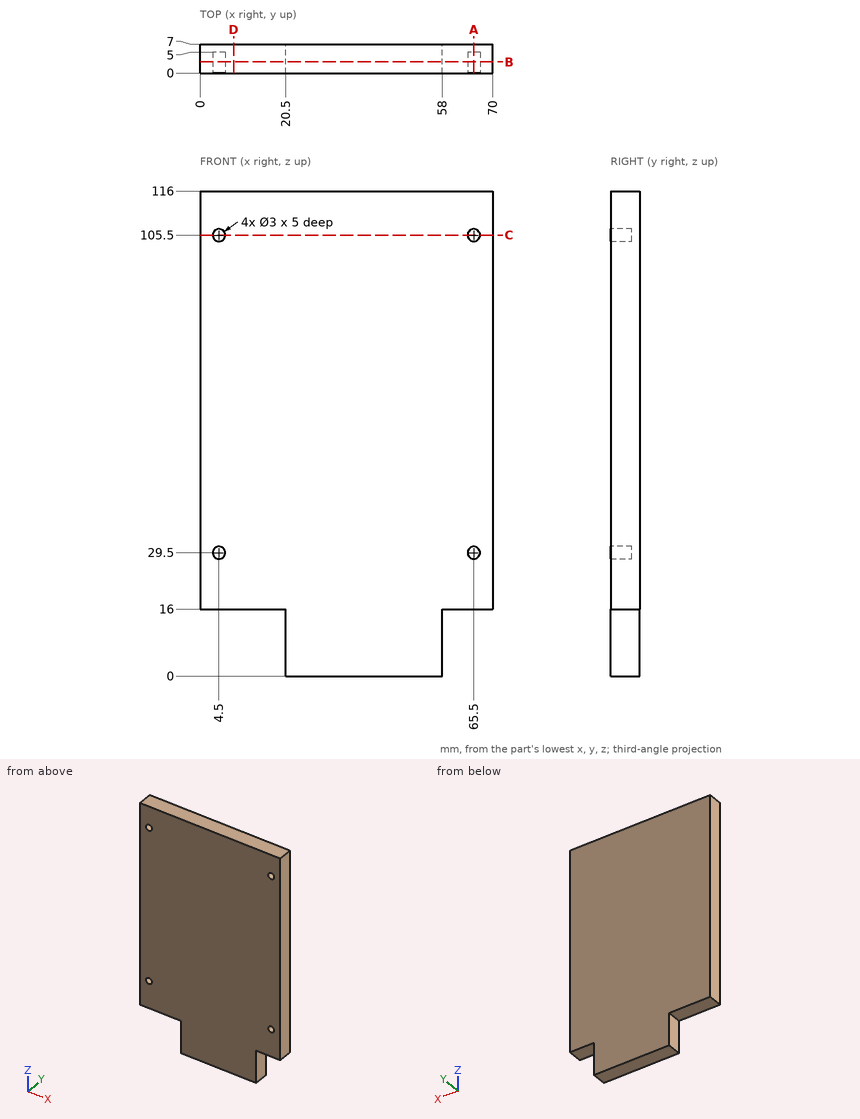
Could you check a few things on this drawing? It's one solid part, dimensions in mm from its lowest x, y, z. Coordinates: 2 decimals unless noted, no trailing zeros. Order: outer loops, then holes, each group sorted by start corner. A loop starts at its lowest first (then second) coordinate and runs counter-clockwise, first axis right, second up. Notation, with made-up numbers: (-34, 84) - (10, 84) arc R32 ccw to (10, 118) - close; hole circle Ø9 at (-16, -14.75). An arc over 180 degrees is marked (long way). One line per question, with ' | ' between items.
(1) If I drill on L1, parallel to X at y = 1.65, z = 29.5; L2, parallel to Z at x = 65.5, y = 3.05; L3, parallel to X at y = 3, z = 104.5, over which ranges is the centre line in solid material (lowest first)?
Report:
L1: x = 0 to 3, 6 to 64, 67 to 70 | L2: z = 16 to 28, 31 to 104, 107 to 116 | L3: x = 0 to 3.38, 5.62 to 64.38, 66.62 to 70
(2) Suppose I cut it at B-B on y = 2.75. List the corners of the cut face in (x, z) for me.
Report:
outline: (0, 16) - (20.5, 16) - (20.5, 0) - (58, 0) - (58, 16) - (70, 16) - (70, 116) - (0, 116) - close; hole circle Ø3 at (4.5, 29.5); hole circle Ø3 at (4.5, 105.5); hole circle Ø3 at (65.5, 29.5); hole circle Ø3 at (65.5, 105.5)
(3) Suppose I cut it at A-A on x = 65.5. List the corners of the cut face in (y, z) for me.
Report:
outline: (0, 16) - (7, 16) - (7, 116) - (0, 116) - (0, 107) - (5, 107) - (5, 104) - (0, 104) - (0, 31) - (5, 31) - (5, 28) - (0, 28) - close
(4) Suppose I cut it at C-C on z = 105.5. List the corners of the cut face in (x, y) for me, and give its area (3 significant figures).
Report:
outline: (0, 0) - (3, 0) - (3, 5) - (6, 5) - (6, 0) - (64, 0) - (64, 5) - (67, 5) - (67, 0) - (70, 0) - (70, 7) - (0, 7) - close | area: 460 mm2
(5) Suppose I cut it at D-D on x = 8. List the corners of the cut face in (y, z) for me.
Report:
outline: (0, 16) - (7, 16) - (7, 116) - (0, 116) - close
(6) Will these pins go through, and if not, where does the flat tip stop? pin 1 (2.5 mm diameter, centred on x = 65.5, z = 29.5, fed in from -Y); pin 2 (3.5 mm diameter, centred on y = 3.5, z = 11, fed in from +X).
Report:
pin 1: stops at y = 5 | pin 2: stops at x = 58
